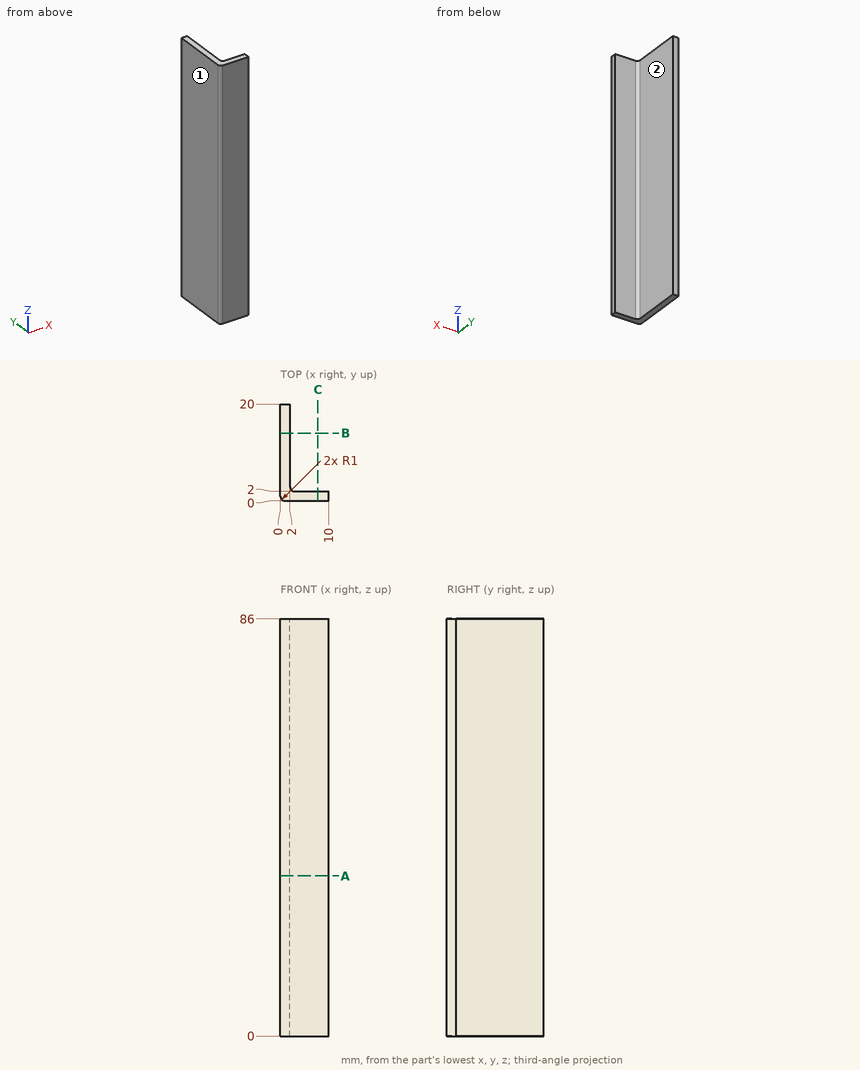
Study the drawing (mm; zero at the part's minimum x, y, z) and answer. A direction names the side the tool comes from. Give positions to 0.01 mm unless a question says otherwise; leave off trailing zeros. Write each loop counter-clockwise with the first axis right and the second up, starting at its lowest first coordinate (ties: lowest second). Pieces come first, ordered by that corner, then holes. Notation, with made-up numbers: (44.25, 14) -> (55.25, 14) arc R19 ccw to (55.25, 36) -> close; hole circle Ø3 at (-25, 11.5). An arc over 180 degrees is marked (long way). Answer as a JSON object with one key per item and string values. Group by question number.
1) Each of these flat-tipped pins is pushed along its axis until it touches: P1, Ø1.5, axis at x = 4, y = 3, coming from the +Z side; P2, Ø5, axis at x = 9, z = 14.5, coming from the +Y side; P3, Ø5, axis at y = 7.5, z = 53, coming from the +X side; P4, Ø1.5, axis at y = 3, z = 77, coming from the +X side. Where does it stop, or does it pass through?
2) Consider L1, parallel to X at y = 8.5, z = 31.5; L2, parallel to Y at x = 0.5, z = 66. Determine where each line is inside the solid, lowest interval first. Write a range as from..to.
3) Find section A-A (z = 33). Write down the section's boundary in (x, y), and give its area (3 significant figures).
4) Find section B-B (y = 14). Write down the section's boundary in (x, z).
5) A tool of negligible diameter and unlimited length cuts with its end or side. For the marked faces 1 and 2, from which of +Z, -Z, +X, -X, +Y, -Y can it reach the whole face along a straight path? Write none if from no direction.
Values follow:
{
 "1": {"P1": "passes through", "P2": "stops at y = 2", "P3": "stops at x = 2", "P4": "stops at x = 2.34"},
 "2": {"L1": "x = 0..2", "L2": "y = 0.13..20"},
 "3": {"outline": "(0, 1) arc R1 ccw to (1, 0) -> (10, 0) -> (10, 2) -> (3, 2) arc R1 cw to (2, 3) -> (2, 20) -> (0, 20) -> close", "area": "56.0 mm2"},
 "4": {"outline": "(0, 0) -> (2, 0) -> (2, 86) -> (0, 86) -> close"},
 "5": {"face 1": "+Z, -Z, -X, +Y, -Y", "face 2": "+Z, -Z, +X, +Y"}
}
